Read the model definition and answer for the solid it produces. Units are mm, in the model's axes. A direction names the side the tool comes from. Round coordinates to 2 decimals unless told otherwise and drop trailing zeros. Order: outer loops, then holes, each group sorted by start corner. A loop starts at its lowest first (then second) coordinate and runs counter-clockwise, first axis right, second up. Notation, with made-up numbers: (31.25, 14) - (51.25, 14) arc R12 cw to (51.25, 37) - close; hole circle Ø6 at (-0.75, 6). An arc over 180 degrees is marked (long way). Put each result on its own line as item: value. Start each with the question number.
Q1. Section A-A on y = 8 is taken. Give the vertices of the cut face in (x, z), then the cut area to 3 significant figures.
Q2. Each of these flat-tipped pins is pushed along its axis until it touches: pin 1 Ø1.2 at (x, y) = (8, -8.5) entering from +Z; pin 2 Ø4 at (x, y) = (-8, -8) entering from +Z; pin 3 Ø2 at (x, y) = (5.5, -2.5) entering from +Z. Where does it stop, or does it pass through?
Q3. For a pull along Y with two mould halves and no side action, classify faces 3 (the face through (-9.815, -9.799, -15.21)), 4 (the face through (8, 8, -3.5)), 5 (the face through (0, 0, 15)) as pulls with the +Y half, pulls with the -Y half, needs draft (parallel to the pull), parting line crosses it, or undercut.
Q4. Section D-D on x = 3 is taken. Give the vertices of the cut face in (y, z), then the cut area to 3 significant figures.
Q5. Find the intervals of material crossed by line 1 along Y through (x, z) = (8, -1.5); line 2 along Z through (x, y) = (-3, -3); line 3 along Z through (x, y) = (6.5, -7.25), in increasing order. Write a range as from..to.
Q6. Which of the six approach directions +Z, -Z, +X, -X, +Y, -Y give full straight-line access (tool end or side, diameter ignored) to faces 1 (the face through (0, -2, 8)), 2 (the face through (-10.1, 0, -15))?
Q7. Section B-B on z = -1 is taken. Give the vertices of the cut face in (x, y), then the cut area to 3 significant figures.
from build123d import *

# Parameters (mm, degrees)
ESQUISSE1_W             = 20.2
ESQUISSE1_H             = 20.2
BOSS_EXTRU_1_DEPTH      = 30
ESQUISSE2_R             = 7.5
BOSS_EXTRU_2_DEPTH      = 1.5
ESQUISSE3_R             = 2
BOSS_EXTRU_4_DEPTH      = 13.5
ESQUISSE4_R             = 1.2
ENL_V_MAT_EXTRU_1_DEPTH = 3.5
CONG_1_R                = 1


with BuildPart() as part:
    # Esquisse1 → Boss.-Extru.1 (new body)
    with BuildSketch(Plane.XY):
        Rectangle(ESQUISSE1_W, ESQUISSE1_H)
    extrude(amount=-BOSS_EXTRU_1_DEPTH)

    # Esquisse2 → Boss.-Extru.2 (add)
    with BuildSketch(Plane.XY):
        Circle(ESQUISSE2_R)
    extrude(amount=BOSS_EXTRU_2_DEPTH)

    # Esquisse3 → Boss.-Extru.4 (add)
    with BuildSketch(Plane.XY.offset(1.5)):
        Circle(ESQUISSE3_R)
    extrude(amount=BOSS_EXTRU_4_DEPTH)

    # Esquisse4 → Enlèv. mat.-Extru.1 (cut)
    with BuildSketch(Plane.XY):
        with Locations((-8, 8)):
            Circle(ESQUISSE4_R)
        with Locations((8, 8)):
            Circle(ESQUISSE4_R)
        with Locations((8, -8)):
            Circle(ESQUISSE4_R)
        with Locations((-8, -8)):
            Circle(ESQUISSE4_R)
    extrude(amount=-ENL_V_MAT_EXTRU_1_DEPTH, mode=Mode.SUBTRACT)

    # Congé1
    cong_1_edges = [part.edges().sort_by_distance(p)[0] for p in [
        (-10.1, 10.1, -15),
        (10.1, 10.1, -15),
        (10.1, -10.1, -15),
        (-10.1, -10.1, -15),
    ]]
    fillet(cong_1_edges, radius=CONG_1_R)


solid = part.part
Findings:
1. outline: (-10.1, -30) - (10.1, -30) - (10.1, 0) - (9.2, 0) - (9.2, -3.5) - (6.8, -3.5) - (6.8, 0) - (-6.8, 0) - (-6.8, -3.5) - (-9.2, -3.5) - (-9.2, 0) - (-10.1, 0) - close
1. area: 589 mm2
2. pin 1: z = -3.5
2. pin 2: z = 0
2. pin 3: z = 1.5
3. face 3: pulls with the -Y half
3. face 4: undercut
3. face 5: needs draft
4. outline: (-10.1, -30) - (10.1, -30) - (10.1, 0) - (6.87, 0) - (6.87, 1.5) - (-6.87, 1.5) - (-6.87, 0) - (-10.1, 0) - close
4. area: 627 mm2
5. line 1: -10.1..-9.2, -6.8..6.8, 9.2..10.1
5. line 2: -30..1.5
5. line 3: -30..0
6. face 1: +Z
6. face 2: +Z, -Z, -X, +Y, -Y
7. outline: (-10.1, -9.1) arc R1 ccw to (-9.1, -10.1) - (9.1, -10.1) arc R1 ccw to (10.1, -9.1) - (10.1, 9.1) arc R1 ccw to (9.1, 10.1) - (-9.1, 10.1) arc R1 ccw to (-10.1, 9.1) - close; hole circle Ø2.4 at (-8, -8); hole circle Ø2.4 at (-8, 8); hole circle Ø2.4 at (8, -8); hole circle Ø2.4 at (8, 8)
7. area: 389 mm2
